Here's how the part is built. I have some questions about the finished solid (model axes, mm). Round coordinates to 2 decimals unless told otherwise and drop trailing zeros. Loops run counter-clockwise (first coordinate to the right, second up) from the corner with the lowest first, then second, coordinate; pieces in that order, holes last. Notation, with made-up numbers: (48.25, 48.25) - (91.25, 48.25) arc R34 cw to (91.25, 84.25) - close; hole circle Ø6 at (89, -29.75). An arc over 180 degrees is marked (long way). Return JSON: item names as keys, results as strings. Group by question number.
```python
from build123d import *

# Parameters (mm, degrees)
BOSS_EXTRUDE1_DEPTH            = 12.7
SKETCH2_R                      = 3.96875
CUT_EXTRUDE1_DEPTH             = 13.7
FILLET1_R                      = 6.35
SKETCH4_R                      = 3.937
CUT_EXTRUDE2_DEPTH             = 13.7
F_5_16_0_3125_DIAMETER_HOLE1_D = 7.9375


with BuildPart() as part:
    # Sketch1 → Boss-Extrude1 (new body)
    with BuildSketch(Plane.XY):
        with BuildLine():
            Line((63.5, 0), (63.5, 120.65))
            Line((63.5, 120.65), (458.219565432, 88.85900811))
            ThreePointArc((458.219565432, 88.85900811), (466.533768826, 84.812244743), (469.9, 76.2))
            Line((469.9, 76.2), (469.9, 0))
            Line((469.9, 0), (63.5, 0))
        make_face()
    extrude(amount=BOSS_EXTRUDE1_DEPTH)

    # Sketch2 → Cut-Extrude1 (cut, through all)
    with BuildSketch(Plane.XY.offset(12.7)):
        with Locations((127, 12.7)):
            Circle(SKETCH2_R)
        with Locations((381, 12.7)):
            Circle(SKETCH2_R)
    extrude(amount=-CUT_EXTRUDE1_DEPTH, mode=Mode.SUBTRACT)

    # Fillet1
    fillet1_edges = [part.edges().sort_by_distance(p)[0] for p in [
        (469.9, 0, 6.35),
    ]]
    fillet(fillet1_edges, radius=FILLET1_R)

    # Sketch4 → Cut-Extrude2 (cut, through all)
    with BuildSketch(Plane(origin=(0, 0, 0), x_dir=(-1, 0, 0), z_dir=(0, 0, -1))):
        with Locations((-416.56762, 76.2)):
            Circle(SKETCH4_R)
        with Locations((-416.56762, 19.05)):
            Circle(SKETCH4_R)
    extrude(amount=-CUT_EXTRUDE2_DEPTH, mode=Mode.SUBTRACT)

    # 5/16 (0.3125) Diameter Hole1 (through all)
    with Locations(Plane.XY.offset(12.7)):
        with Locations((334.9625, 14.2875), (334.9625, 68.2625)):
            Hole(F_5_16_0_3125_DIAMETER_HOLE1_D / 2)


solid = part.part
```
Q1. If we mould it in two halves opening along Y, with no side actions, what happens to faces 1 (the cylindrical face through (420.5, 19.2, 6.3)), 2 (the cylindrical face through (466.44, 84.91, 6.26)), 3 (the flat face through (63.5, 59, 6)), 4 (the cylindrical face through (331.177, 69.455, 6.261))? For each: +Y half, -Y half, draft (parallel to the pull), parting line (faces both ways), or undercut.
Q2. Will these pins go through, and if not, where does the flat tip stop? pin 1 Ø9 at (x, y) = (416.57, 19.05) entering from +Z; pin 2 Ø1.5 at (x, z) = (120, 5.5) entering from +Y.
Q3. Imagine slicing it at B-B, the plane z = 3.5. List the corners of the cut face in (x, y) for me, and give its area (3 significant figures).
Q4. Imagine slicing it at A-A, the plane x = 381. List the corners of the cut face in (y, z) for me.
Q5. Imagine slicing it at C-C, the plane x = 127. List the corners of the cut face in (y, z) for me, and give its area (3 significant figures).
Q6. Please list where these lines run through material, in increasing order: line 1 (X direction, y = 14.5, z = 10.25); line 2 (X direction, y = 76, z = 7); line 3 (Y direction, x = 381, z = 3).
Q7. Imagine slicing it at D-D, the plane x = 327. List the corners of the cut face in (y, z) for me.
Output values:
{
 "1": {"face 1": "undercut", "face 2": "+Y half", "face 3": "draft", "face 4": "undercut"},
 "2": {"pin 1": "stops at z = 12.7", "pin 2": "stops at y = 116.16"},
 "3": {"outline": "(63.5, 0) - (463.55, 0) arc R6.35 ccw to (469.9, 6.35) - (469.9, 76.2) arc R12.7 ccw to (458.22, 88.86) - (63.5, 120.65) - close; hole circle Ø7.94 at (127, 12.7); hole circle Ø7.94 at (334.96, 14.29); hole circle Ø7.94 at (334.96, 68.26); hole circle Ø7.94 at (381, 12.7); hole circle Ø7.87 at (416.57, 19.05); hole circle Ø7.87 at (416.57, 76.2)", "area": "42,000 mm^2"},
 "4": {"outline": "(0, 0) - (8.73, 0) - (8.73, 12.7) - (0, 12.7) - close; (16.67, 0) - (95.08, 0) - (95.08, 12.7) - (16.67, 12.7) - close"},
 "5": {"outline": "(0, 0) - (8.73, 0) - (8.73, 12.7) - (0, 12.7) - close; (16.67, 0) - (115.54, 0) - (115.54, 12.7) - (16.67, 12.7) - close", "area": "1,370 mm^2"},
 "6": {"line 1": "x = 63.5 to 123.46, 130.54 to 331, 338.93 to 377.46, 384.54 to 469.9", "line 2": "x = 63.5 to 412.64, 420.5 to 469.9", "line 3": "y = 0 to 8.73, 16.67 to 95.08"},
 "7": {"outline": "(0, 0) - (99.43, 0) - (99.43, 12.7) - (0, 12.7) - close"}
}
